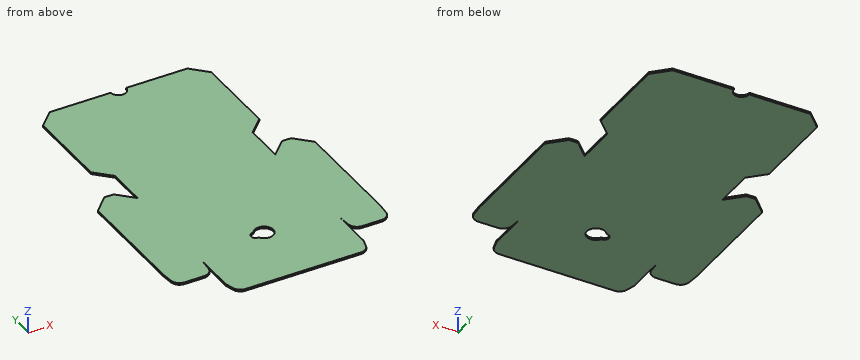
from build123d import *

# Parameters (mm, degrees)
F1_DEPTH = 1.23
F3_DEPTH = 1.231


with BuildPart() as f1:
    # F0 (on Top) → F1 (new body)
    with BuildSketch(Plane.XY):
        Polygon((-70.759976, 27.804737), (-70.759976, -47.195263), (-70.101805, -54.718197), (-69.920191, -55.748177), (-69.562483, -56.730973), (-69.039549, -57.636722), (-68.367277, -58.437904), (-67.566095, -59.110175), (-66.660346, -59.63311), (-65.677551, -59.990818), (-64.647571, -60.172431), (-64.124636, -60.195263), (-51.395316, -60.195263), (-50.353427, -60.10411), (-49.343195, -59.833419), (-48.395316, -59.391415), (-47.53859, -58.79153), (-46.799049, -58.051989), (-46.199163, -57.195263), (-45.75716, -56.247384), (-45.486469, -55.237152), (-45.418147, -54.718197), (-44.759976, -47.195263), (-44.759976, -73.195263), (-43.272077, -78.748177), (-42.914369, -79.730973), (-42.391434, -80.636722), (-41.719163, -81.437904), (-40.917981, -82.110175), (-40.012232, -82.63311), (-39.029436, -82.990818), (-37.999457, -83.172431), (-37.476522, -83.195263), (37.95657, -83.195263), (38.998459, -83.10411), (40.008691, -82.833419), (40.95657, -82.391415), (41.813296, -81.79153), (42.552837, -81.051989), (43.152723, -80.195263), (43.594726, -79.247384), (43.752125, -78.748177), (45.240024, -73.195263), (45.240024, -47.195263), (45.898195, -54.718197), (46.079809, -55.748177), (46.437517, -56.730973), (46.960451, -57.636722), (47.632723, -58.437904), (48.433905, -59.110175), (49.339654, -59.63311), (50.322449, -59.990818), (51.352429, -60.172431), (51.875364, -60.195263), (64.604684, -60.195263), (65.646573, -60.10411), (66.656805, -59.833419), (67.604684, -59.391415), (68.46141, -58.79153), (69.200951, -58.051989), (69.800837, -57.195263), (70.24284, -56.247384), (70.513531, -55.237152), (70.581853, -54.718197), (71.240024, -47.195263), (71.240024, 27.804737), (61.240024, 37.804737), (55.240024, 37.804737), (45.240024, 27.804737), (45.240024, 53.804737), (55.240024, 63.804737), (55.240024, 118.804737), (45.240024, 128.804737), (5.240024, 128.804737), (5.164063, 127.936496), (4.938487, 127.094636), (4.570151, 126.304737), (4.070246, 125.590799), (3.453962, 124.974515), (2.740024, 124.47461), (1.950125, 124.106274), (1.108265, 123.880698), (0.240024, 123.804737), (-0.628217, 123.880698), (-1.470077, 124.106274), (-2.259976, 124.47461), (-2.973914, 124.974515), (-3.590198, 125.590799), (-4.090103, 126.304737), (-4.458439, 127.094636), (-4.684015, 127.936496), (-4.759976, 128.804737), (-44.759976, 128.804737), (-54.759976, 118.804737), (-54.759976, 63.804737), (-44.759976, 53.804737), (-44.759976, 27.804737), (-54.759976, 37.804737), (-60.759976, 37.804737), align=None)
    extrude(amount=F1_DEPTH)

    # F2 (on face) → F3 (cut, through all)
    with BuildSketch(Plane.XY.offset(1.23)):
        with BuildLine():
            ThreePointArc((-4.964521, -35.209847), (-8.259976, -38.195263), (-4.964521, -41.180679))
            ThreePointArc((-4.964521, -41.180679), (6.240024, -38.195263), (-4.964521, -35.209847))
        make_face()
    extrude(amount=-F3_DEPTH, mode=Mode.SUBTRACT)


solid = f1.part
Could you check a few things on this model? Use its own coordinates, in mm. Give positions to 0.01 mm unless a question says otherwise; leave off trailing zeros. Write each loop counter-clockwise with the first axis right and the second up, starting at its lowest first coordinate (ties: lowest second). Pieces come first, ordered by that corner, then holes. Notation, with made-up numbers: (-29, -2) -> (12, -2) arc R13 ccw to (12, 22) -> close; hole circle Ø1 at (27.5, 6.5). An arc over 180 degrees is marked (long way). Answer as a JSON object with one key per item and string values.
Q1. Will these pins go through, and if not, where does the flat tip stop? pin 1 Ø0.6 at (y, z) = (-65, 1) entering from -X; pin 2 Ø0.6 at (y, z) = (-64, 1) entering from +X; pin 3 Ø7 at (x, y) = (0.24, -38.2) entering from +Z; pin 4 Ø0.6 at (x, z) = (57, 1) entering from +Y.
Taken from the geometry:
{"pin 1": "stops at x = -44.76", "pin 2": "stops at x = 45.24", "pin 3": "passes through", "pin 4": "stops at y = 37.8"}
Q2. Suppose I cut it at A-A on y = 41.5. Write out the boundary of the cut face in (x, z), then the cut area to 3 significant figures.
Taken from the geometry:
{"outline": "(-44.76, 0) -> (45.24, 0) -> (45.24, 1.23) -> (-44.76, 1.23) -> close", "area": "111 mm²"}
Q3. Please list where these lines run through material, in increasing order: L1, parallel to X at y = 33, z = 0.75; L2, parallel to X at y = -54, z = 0.5; L3, parallel to X at y = 47, z = 0.35.
Taken from the geometry:
{"L1": "x = -65.56 to -49.96, -44.76 to 45.24, 50.44 to 66.04", "L2": "x = -70.16 to -45.36, -44.76 to 45.24, 45.84 to 70.64", "L3": "x = -44.76 to 45.24"}
Q4. Suppose I cut it at B-B on y = 83.5. Write out the boundary of the cut face in (x, z), then the cut area to 3 significant figures.
Taken from the geometry:
{"outline": "(-54.76, 0) -> (55.24, 0) -> (55.24, 1.23) -> (-54.76, 1.23) -> close", "area": "135 mm²"}
